Could you check a few things on this model? Use its own coordinates, in mm. A direction names the side the tool comes from. Give positions to 0.01 mm unless a question says otherwise; leave off trailing zeros. Order: outer loops, then holes, each group sorted by start corner. A loop starts at its lowest first (then second) coordinate and runs counter-clockwise, first axis right, second up.
(1) Imagine slicing it at B-B, the plane z = 8.25. Write out the boundary of the cut face in (x, y).
(2) If we mould it in two halves opening along Y, with no side actions, what happens to faces 4 (the cylindrical face through (-27, -12.9, 6.6)), 5 (the flat face through (22, -10, 5)), 6 (the flat face through (2, 12, 13))? For each: released by +Y, released by -Y, zero draft, split by the parting line, or undercut.
(3) On a 3-axis mill with a long thin cutter (end or side, diameter ignored), from which of +Z, -Z, +X, -X, +Y, -Y can I reach the whole of each face in a straight line? I mean faces 1 (the flat face through (24, -6.14, 4)), 2 (the cylindrical face through (26.9, -13, 6.6)), 3 (the flat face through (25.4, 0, 8)). Say none if no direction works.
(4) If I drill on probe 1 along Y at (x, z) = (-22.86, 4.45); probe 2 along Y at (x, z) = (-22.86, 1.3); probe 3 along Y at (x, z) = (21, 5.75), over which ranges is the centre line in solid material (lowest first)?
(5) Imagine slicing it at A-A, the plane z = 1. Write out the boundary of the cut face in (x, y), then the cut area to 3 significant figures.
(6) Will these pins go through, and if not, where does the flat tip stop? pin 1 (2.5 mm diameter, centred on x = -23, y = -8, fed in from +Z); pin 2 (11.5 mm diameter, centred on x = -14.5, y = -5.5, fed in from +Z); pin 3 (3 mm diameter, centred on x = -25.5, z = 6, fed in from -Y).
(7) Imagine slicing it at D-D, the plane y = -3.75. Write out the boundary of the cut face in (x, z).
(8) Imagine slicing it at C-C, the plane x = 14. Write out the boundary of the cut face in (y, z).
from build123d import *

# Parameters (mm, degrees)
F0_W      = 56.8
F0_H      = 28.86
F1_DEPTH  = 3
F2_W      = 56.8
F2_H      = 28.86
F2_W_2    = 50.8
F2_H_2    = 22.86
F3_DEPTH  = 10
F4_W      = 5.29
F4_H      = 5.29
F4_R      = 1.25
F5_DEPTH  = 2
F6_R      = 2.75
F7_R      = 2
F8_R      = 5
F9_W      = 12.28
F9_H      = 10
F10_DEPTH = 3
F11_DEPTH = 3


with BuildPart() as f1:
    # F0 (on Top) → F1 (new body)
    with BuildSketch(Plane.XY):
        Rectangle(F0_W, F0_H)
    extrude(amount=F1_DEPTH)

    # F2 (on face) → F3 (join)
    with BuildSketch(Plane.XY.offset(3)):
        Rectangle(F2_W, F2_H)
        Rectangle(F2_W_2, F2_H_2, mode=Mode.SUBTRACT)
    extrude(amount=F3_DEPTH)

    # F4 (on face) → F5 (join)
    with BuildSketch(Plane.XY.offset(3)):
        with Locations((-22.755, 8.785)):
            Rectangle(F4_W, F4_H)
        with Locations((-22.86, 8.89)):
            Circle(F4_R, mode=Mode.SUBTRACT)
        with Locations((22.755, -8.785)):
            Rectangle(F4_W, F4_H)
        with Locations((22.86, -8.89)):
            Circle(F4_R, mode=Mode.SUBTRACT)
        with Locations((22.755, 8.785)):
            Rectangle(F4_W, F4_H)
        with Locations((22.86, 8.89)):
            Circle(F4_R, mode=Mode.SUBTRACT)
        with Locations((-22.755, -8.785)):
            Rectangle(F4_W, F4_H)
        with Locations((-22.86, -8.89)):
            Circle(F4_R, mode=Mode.SUBTRACT)
    extrude(amount=F5_DEPTH)

    # F6
    f6_edges = [f1.edges().sort_by_distance(p)[0] for p in [
        (-20.11, 6.14, 4),
        (20.11, 6.14, 4),
        (20.11, -6.14, 4),
        (-20.11, -6.14, 4),
    ]]
    fillet(f6_edges, radius=F6_R)

    # F7
    f7_edges = [f1.edges().sort_by_distance(p)[0] for p in [
        (-25.4, 11.43, 9),
        (25.4, 11.43, 9),
        (25.4, -11.43, 9),
        (-25.4, -11.43, 9),
    ]]
    fillet(f7_edges, radius=F7_R)

    # F8
    f8_edges = [f1.edges().sort_by_distance(p)[0] for p in [
        (28.4, 14.43, 6.5),
        (28.4, -14.43, 6.5),
        (-28.4, -14.43, 6.5),
        (-28.4, 14.43, 6.5),
    ]]
    fillet(f8_edges, radius=F8_R)

    # F9 (on face) → F10 (cut, through all)
    with BuildSketch(Plane.YZ.offset(-25.4)):
        with Locations((0, 8)):
            Rectangle(F9_W, F9_H)
    extrude(amount=-F10_DEPTH, mode=Mode.SUBTRACT)

    # F11 (cut, through all): faces of the model
    f11_faces = [f1.faces().sort_by_distance(p)[0] for p in [
        (22.86, 8.89, 3),
        (22.86, -8.89, 3),
        (-22.86, -8.89, 3),
        (-22.86, 8.89, 3),
    ]]
    extrude(f11_faces, amount=-F11_DEPTH, mode=Mode.SUBTRACT)


solid = f1.part
Answer block:
1. outline: (-28.4, -9.43) arc R5 ccw to (-23.4, -14.43) - (23.4, -14.43) arc R5 ccw to (28.4, -9.43) - (28.4, 9.43) arc R5 ccw to (23.4, 14.43) - (-23.4, 14.43) arc R5 ccw to (-28.4, 9.43) - (-28.4, 6.14) - (-25.4, 6.14) - (-25.4, 9.43) arc R2 cw to (-23.4, 11.43) - (23.4, 11.43) arc R2 cw to (25.4, 9.43) - (25.4, -9.43) arc R2 cw to (23.4, -11.43) - (-23.4, -11.43) arc R2 cw to (-25.4, -9.43) - (-25.4, -6.14) - (-28.4, -6.14) - close
2. face 4: released by -Y
2. face 5: undercut
2. face 6: zero draft
3. face 1: +Z, -X
3. face 2: +Z, -Z, +X, -Y
3. face 3: +Z
4. probe 1: y = -14.43 to -10.14, -7.64 to -6.14, 6.14 to 7.64, 10.14 to 14.43
4. probe 2: y = -14.43 to -10.14, -7.64 to 7.64, 10.14 to 14.43
4. probe 3: y = -14.43 to -11.43, 11.43 to 14.43
5. outline: (-28.4, -9.43) arc R5 ccw to (-23.4, -14.43) - (23.4, -14.43) arc R5 ccw to (28.4, -9.43) - (28.4, 9.43) arc R5 ccw to (23.4, 14.43) - (-23.4, 14.43) arc R5 ccw to (-28.4, 9.43) - close; hole circle Ø2.5 at (-22.86, -8.89); hole circle Ø2.5 at (-22.86, 8.89); hole circle Ø2.5 at (22.86, -8.89); hole circle Ø2.5 at (22.86, 8.89)
5. area: 1,600 mm2
6. pin 1: stops at z = 5
6. pin 2: stops at z = 3
6. pin 3: stops at y = -14.39
7. outline: (-28.4, 0) - (28.4, 0) - (28.4, 13) - (25.4, 13) - (25.4, 3) - (-28.4, 3) - close
8. outline: (-14.43, 0) - (14.43, 0) - (14.43, 13) - (11.43, 13) - (11.43, 3) - (-11.43, 3) - (-11.43, 13) - (-14.43, 13) - close
